Autodesk Fusion 360 part; units mm, degrees
sketch "Sketch1" plane through (0, 0, 0) normal (0, 1, 0) x (1, 0, 0)
  circle A0 centre (0, 0) radius 26.5
  circle A1 centre (0, 0) radius 40
  dimension "d1" = 53
  dimension "d2" = 80
extrude "Extrude1" add sketch "Sketch1" along normal blind 15 contours A0
extrude "Extrude2" add sketch "Sketch1" against normal blind 6 contours A0 | A1
sketch "Sketch2" plane through (0, 15, 0) normal (0, 1, 0) x (-1, 0, 0)
  circle A0 centre (0, 0) radius 26.5
  circle A1 centre (0, 0) radius 15.125
  dimension "d7" = 30.25
extrude "Extrude3" cut sketch "Sketch2" against normal blind 77.834 contours A1
sketch "Sketch3" plane through (0, 15, 0) normal (0, 1, 0) x (-1, 0, 0)
  circle A0 centre (0, 0) radius 15.125
  circle A1 centre (0, 0) radius 26.5
  circle A2 centre (0, 0) radius 21.5
  dimension "d10" = 43
extrude "Extrude4" cut sketch "Sketch3" against normal blind 9 contours A2
chamfer "Chamfer1" distance 2 angle 45 1 edges at (14.1015, -6, -5.4694)
Geometry: final body of the model. Coordinates: model frame, mm. A direction names the side the tool comes from. Round coordinates to 2 decimals unless told otherwise and drop trailing zeros. Write each loop counter-clockwise with the first axis right and the second up, starting at its lowest first coordinate (ties: lowest second). Pieces come first, ordered by that corner, then holes.
Item 1: Set-up query: faces 5 (the face through (3.279, 1.07, -14.765)), 6 (the face through (-4, 6, 15)). Return all of +Z, -Z, +X, -X, +Y, -Y with unobstructed straight access to the full face (end or side cutting, diameter ignored); none if empty.
Item 2: Section query B-B (z = 0). Return loops of the section in (x, y) (3 decimals), plus the area to 3 significant figures.
Item 3: Section query C-C (y = 2.5). Return loops of the section in (x, z) (3 decimals), plus the area to 3 significant figures.
Item 4: Mould query, pull axis Z, two halves, no side actions, for faces 1 (the face through (3.31, -4.13, 14.89)), 2 (the face through (-8.67, -2.96, 39.05)), 3 (the face through (2.799, 10.563, 21.317)), 4 (the face through (0, 15, -22)). Classes: +Z half, -Z half, draft (parallel to the pull), parting line (faces both ways), or undercut.
Item 5: Section query A-A (x = 0). Return loops of the section in (y, z) (3 decimals), plus the area to 3 significant figures.
Item 6: Section query D-D (z = -23.5). Return loops of the section in (x, y).
Item 7: Material intervals for L1, parallel to Z at x = 0, y = 11.25; L2, parallel to Y at x = 30, z = 21.5; L3, parallel to Z at x = 0, y = -1 (3 decimals), sorted ascending.
Item 8: Pin query (flat end, axial travel): P1, Ø10, axis at y = 3, z = 17, coming from the -X side; P2, Ø5, axis at x = -19.5, y = 9.5, coming from the +Z side; P3, Ø8, axis at y = 1, z = -23, coming from the +X side; P4, Ø24, axis at x = 0, z = 0, coming from the -Y side. Return the tip coordinate at first contact, or that it passes through.
Completed:
1. face 5: +Y, -Y
1. face 6: +Y
2. outline: (-40, -6) - (-17.125, -6) - (-15.125, -4) - (-15.125, 6) - (-21.5, 6) - (-21.5, 15) - (-26.5, 15) - (-26.5, 0) - (-40, 0) - close; (15.125, -4) - (17.125, -6) - (40, -6) - (40, 0) - (26.5, 0) - (26.5, 15) - (21.5, 15) - (21.5, 6) - (15.125, 6) - close
2. area: 521 mm2
3. outline: circle Ø53 at (0, 0); hole circle Ø30.25 at (0, 0)
3. area: 1,490 mm2
4. face 1: undercut
4. face 2: parting line
4. face 3: undercut
4. face 4: draft
5. outline: (-6, -40) - (0, -40) - (0, -26.5) - (15, -26.5) - (15, -21.5) - (6, -21.5) - (6, -15.125) - (-4, -15.125) - (-6, -17.125) - close; (-6, 17.125) - (-4, 15.125) - (6, 15.125) - (6, 21.5) - (15, 21.5) - (15, 26.5) - (0, 26.5) - (0, 40) - (-6, 40) - close
5. area: 521 mm2
6. outline: (-32.37, -6) - (32.37, -6) - (32.37, 0) - (12.25, 0) - (12.25, 15) - (-12.25, 15) - (-12.25, 0) - (-32.37, 0) - close
7. L1: z = -26.5 to -21.5, 21.5 to 26.5
7. L2: y = -6 to 0
7. L3: z = -40 to -15.125, 15.125 to 40
8. P1: stops at x = -37.83
8. P2: stops at z = 20.33
8. P3: stops at x = 35.13
8. P4: passes through
